```python
from build123d import *

# Parameters (mm, degrees)
SKETCH_R           = 17.85
PAD_DEPTH          = 91.7
SKETCH001_R        = 11
PAD001_DEPTH       = 2
SKETCH002_R        = 3
PAD002_DEPTH       = 13.4
SKETCH003_R        = 1.5
POCKET_DEPTH       = 10
POLARPATTERN_COUNT = 4


with BuildPart() as part:
    # Sketch → Pad (new body)
    with BuildSketch(Plane.YZ):
        Circle(SKETCH_R)
    extrude(amount=PAD_DEPTH)

    # Sketch001 → Pad001 (join)
    with BuildSketch(Plane.YZ):
        Circle(SKETCH001_R)
    extrude(amount=-PAD001_DEPTH)

    # Sketch002 (on Face5 of Pad001) → Pad002 (join)
    with BuildSketch(Plane(origin=(-2, 0, 0), x_dir=(0, -1, 0), z_dir=(-1, 0, 0))):
        Circle(SKETCH002_R)
    extrude(amount=PAD002_DEPTH)

    # Sketch003 → Pocket (cut)
    with BuildSketch(Plane.YZ):
        with Locations((0, 14)):
            Circle(SKETCH003_R)
    pocket = extrude(amount=POCKET_DEPTH, mode=Mode.SUBTRACT)

    # PolarPattern: Pocket ×4 about axis
    polarpattern_axis = Axis((0, 0, 0), (1, 0, 0))
    for i in range(1, POLARPATTERN_COUNT):
        add(pocket.rotate(polarpattern_axis, i * 360 / POLARPATTERN_COUNT), mode=Mode.SUBTRACT)


solid = part.part
```
The model under review builds one solid part; all positions refer to its coordinate system, in mm. A direction names the side the tool comes from. Round coordinates to 2 decimals unless told otherwise and drop trailing zeros. Loops run counter-clockwise (first coordinate to the right, second up) from the corner with the lowest first, then second, coordinate; pieces in that order, holes last. Notation, with made-up numbers: (61, 46) -> (106, 46) arc R12 ccw to (106, 61) -> close; hole circle Ø2 at (77.5, 25). An arc over 180 degrees is marked (long way). Answer in a Markdown table with one row per item.
1) Consider section C-C, the plane y = -14. Write out the cut boundary in (x, z).
Taken from the geometry:
| item | result |
|---|---|
| outline | (0, -11.07) -> (91.7, -11.07) -> (91.7, 11.07) -> (0, 11.07) -> (0, 1.5) -> (10, 1.5) -> (10, -1.5) -> (0, -1.5) -> close |
2) Tool access review of faces 1 (the cylindrical face through (4.93, 0.325, -12.536)), 2 (the cylindrical face through (45.208, -17.833, 0.785)): name each direction out of +Z, -Z, +X, -X, +Y, -Y from which nothing blocks a thin tool from reaching the whole face with its end or side.
Taken from the geometry:
| item | result |
|---|---|
| face 1 | -X |
| face 2 | +X, -X |
3) Draft analysis for pull direction Y (two halves, no side actions). For faces 3 (the cylindrical face through (-9, 3, 0)), 4 (the flat face through (10, 0, 14)), 5 (the flat face through (-2, 2.3, -2.3)), state which applies: pulls with the +Y half, pulls with the -Y half, needs draft (parallel to the pull), parting line crosses it, or undercut.
Taken from the geometry:
| item | result |
|---|---|
| face 3 | parting line crosses it |
| face 4 | undercut |
| face 5 | needs draft |
4) Consider section B-B, the plane x = 58. Write out the cut boundary in (y, z), plus the area to 3 significant figures.
Taken from the geometry:
| item | result |
|---|---|
| outline | circle Ø35.7 at (0, 0) |
| area | 1,000 mm² |
5) Consider section D-D, the plane z = -6.5. Write out the cut boundary in (x, y), plus the area to 3 significant figures.
Taken from the geometry:
| item | result |
|---|---|
| outline | (-2, -8.87) -> (0, -8.87) -> (0, -16.62) -> (91.7, -16.62) -> (91.7, 16.62) -> (0, 16.62) -> (0, 8.87) -> (-2, 8.87) -> close |
| area | 3,080 mm² |
6) For pin 1 Ø4 at (y, z) = (-14, 0) entering from -X; pin 2 Ø8 at (x, y) = (15, -4.5) entering from -Z; pin 3 Ø0.9 at (y, z) = (0, -14) entering from -X, all flat-tipped, find the tip position at first contact; note any pin that passes through.
Taken from the geometry:
| item | result |
|---|---|
| pin 1 | stops at x = 0 |
| pin 2 | stops at z = -17.84 |
| pin 3 | stops at x = 10 |
7) Wall thickness on line 1 along Z through (x, y) = (6.25, 0); line 2 along X through (y, z) = (7, 2); line 3 along X through (y, z) = (12, 5.5): over which ranges is each line inside the solid? List them lowest first.
Taken from the geometry:
| item | result |
|---|---|
| line 1 | z = -17.85 to -15.5, -12.5 to 12.5, 15.5 to 17.85 |
| line 2 | x = -2 to 91.7 |
| line 3 | x = 0 to 91.7 |
8) Consider section A-A, the plane z = 0. Write out the cut boundary in (x, y).
Taken from the geometry:
| item | result |
|---|---|
| outline | (-15.4, -3) -> (-2, -3) -> (-2, -11) -> (0, -11) -> (0, -12.5) -> (10, -12.5) -> (10, -15.5) -> (0, -15.5) -> (0, -17.85) -> (91.7, -17.85) -> (91.7, 17.85) -> (0, 17.85) -> (0, 15.5) -> (10, 15.5) -> (10, 12.5) -> (0, 12.5) -> (0, 11) -> (-2, 11) -> (-2, 3) -> (-15.4, 3) -> close |
